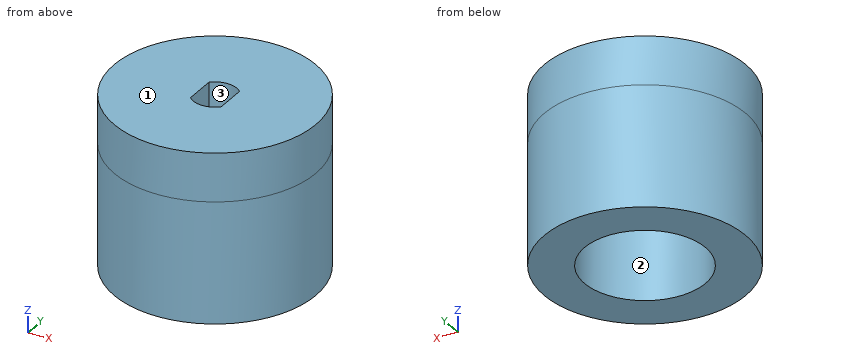
from build123d import *

# Parameters (mm, degrees)
SKETCH2_R           = 25
BOSS_EXTRUDE1_DEPTH = 4
SKETCH3_R           = 25
SKETCH3_R_2         = 1
BOSS_EXTRUDE2_DEPTH = 2
CUT_EXTRUDE1_DEPTH  = 36.860842154
CIRPATTERN1_COUNT   = 30
SKETCH6_R           = 25
SKETCH6_R_2         = 12.5
CUT_EXTRUDE2_DEPTH  = 36.860842154
SKETCH7_R           = 12.5
SKETCH7_R_2         = 7.5
BOSS_EXTRUDE3_DEPTH = 15


with BuildPart() as part:
    # Sketch2 → Boss-Extrude1 (new body)
    with BuildSketch(Plane.XY):
        Circle(SKETCH2_R)
        with BuildLine():
            Line((1.9, -1.918332609), (1.9, 1.918332609))
            ThreePointArc((1.9, 1.918332609), (0, 2.7), (-1.9, 1.918332609))
            Line((-1.9, 1.918332609), (-1.9, -1.918332609))
            ThreePointArc((-1.9, -1.918332609), (0, -2.7), (1.9, -1.918332609))
        make_face(mode=Mode.SUBTRACT)
    extrude(amount=-BOSS_EXTRUDE1_DEPTH)

    # Sketch3 → Boss-Extrude2 (add)
    with BuildSketch(Plane(origin=(0, 0, -4), x_dir=(-1, 0, 0), z_dir=(0, 0, -1))):
        with Locations(Location((0, 0, 0), (0, 0, 180))):
            Circle(SKETCH3_R)
        Circle(SKETCH3_R_2, mode=Mode.SUBTRACT)
    extrude(amount=BOSS_EXTRUDE2_DEPTH)

    # Sketch4 → Cut-Extrude1 (cut, symmetric)
    with BuildSketch(Plane.XY):
        with BuildLine():
            Line((-0.857142857, 18), (0.857142857, 18))
            Line((0.857142857, 18), (0.998868138, 20.976230892))
            ThreePointArc((0.998868138, 20.976230892), (0, 21), (-0.998868138, 20.976230892))
            Line((-0.998868138, 20.976230892), (-0.857142857, 18))
        make_face()
    cut_extrude1 = extrude(amount=CUT_EXTRUDE1_DEPTH, both=True, mode=Mode.SUBTRACT)

    # CirPattern1: Cut-Extrude1 ×30 about axis
    cirpattern1_axis = Axis((0, 0, 0), (0, 0, 1))
    for i in range(1, CIRPATTERN1_COUNT):
        add(cut_extrude1.rotate(cirpattern1_axis, i * 360 / CIRPATTERN1_COUNT), mode=Mode.SUBTRACT)

    # Sketch6 → Cut-Extrude2 (cut, through all)
    with BuildSketch(Plane.XY):
        Circle(SKETCH6_R)
        Circle(SKETCH6_R_2, mode=Mode.SUBTRACT)
    extrude(amount=-CUT_EXTRUDE2_DEPTH, mode=Mode.SUBTRACT)

    # Sketch7 → Boss-Extrude3 (add)
    with BuildSketch(Plane(origin=(0, 0, -6), x_dir=(-1, 0, 0), z_dir=(0, 0, -1))):
        with Locations(Location((0, 0, 0), (0, 0, 180))):
            Circle(SKETCH7_R)
        Circle(SKETCH7_R_2, mode=Mode.SUBTRACT)
    extrude(amount=BOSS_EXTRUDE3_DEPTH)


solid = part.part
The listing builds one solid part. Answer for the finished solid, in the listing's coordinates (mm). Face numbers are marked on the shaded views. Give positions to 0.01 mm unless a question says otherwise; leave off trailing zeros. Loops run counter-clockwise (first coordinate to the right, second up) from the corner with the lowest first, then second, coordinate; pieces in that order, holes last. Notation, with made-up numbers: (84.5, 87.25) - (117.5, 87.25) arc R20 cw to (117.5, 111.25) - close; hole circle Ø6 at (-26.5, 19). An arc over 180 degrees is marked (long way). Write each question's results on one line, items separated by ' | '.
1. Flat-ended cylindrical pins translate along their axes: P1, Ø6, axis at x = -9.5, z = -5, coming from the +Y side; P2, Ø4.5, axis at x = 1.5, y = 3.5, coming from the -Z side; P3, Ø3, axis at x = -5, y = -1, coming from the +Z side; P4, Ø1.5, axis at x = 2.5, z = -18, coming from the -Y side. Find the tip coordinate at first contact, or state that the pin passes through.
Resolved:
P1: stops at y = 10.68 | P2: stops at z = -6 | P3: stops at z = 0 | P4: stops at y = -12.38
2. Find section A-A, the plane y = 0. Write down the section's boundary in (x, z), then the cut area to 3 significant figures.
Resolved:
outline: (-12.5, -21) - (-7.5, -21) - (-7.5, -6) - (-1, -6) - (-1, -4) - (-1.9, -4) - (-1.9, 0) - (-12.5, 0) - close; (1, -6) - (7.5, -6) - (7.5, -21) - (12.5, -21) - (12.5, 0) - (1.9, 0) - (1.9, -4) - (1, -4) - close | area: 281 mm^2
3. Find section C-C, the plane z = -14.5. Write down the section's boundary in (x, y).
Resolved:
outline: circle Ø25 at (0, 0); hole circle Ø15 at (0, 0)
4. For a pull along X with two mould halves and no side action, classify the marked faces 1, 2 and 3 as +X half, -X half, draft (parallel to the pull), parting line (faces both ways), or undercut.
Resolved:
face 1: draft | face 2: undercut | face 3: undercut
5. Find section B-B, the plane x = 0. Write down the section's boundary in (y, z).
Resolved:
outline: (-12.5, -21) - (-7.5, -21) - (-7.5, -6) - (-1, -6) - (-1, -4) - (-2.7, -4) - (-2.7, 0) - (-12.5, 0) - close; (1, -6) - (7.5, -6) - (7.5, -21) - (12.5, -21) - (12.5, 0) - (2.7, 0) - (2.7, -4) - (1, -4) - close
6. Consider probe 1 along Z at (x, y) = (1.25, -7); probe 2 along Y at (x, z) = (0, -10.5); probe 3 along Y at (x, z) = (0, -5.2). Determine where each line is inside the solid, lowest interval first. Write a range as from..to.
Resolved:
probe 1: z = -6..0 | probe 2: y = -12.5..-7.5, 7.5..12.5 | probe 3: y = -12.5..-1, 1..12.5
7. Find section D-D, the plane x = 3. Write down the section's boundary in (y, z), then the cut area to 3 significant figures.
Resolved:
outline: (-12.13, -21) - (-6.87, -21) - (-6.87, -6) - (6.87, -6) - (6.87, -21) - (12.13, -21) - (12.13, 0) - (-12.13, 0) - close | area: 303 mm^2
